Design review of the part built by this model. Coordinates are the model's own, in mm. Face numbers are marked on the shaded views. A direction names the side the tool comes from. Give positions to 0.01 mm unless a question says otherwise; leave off trailing zeros. Write each loop counter-clockwise with the first axis right and the second up, starting at its lowest first coordinate (ties: lowest second). Pieces come first, ordered by that corner, then holes.
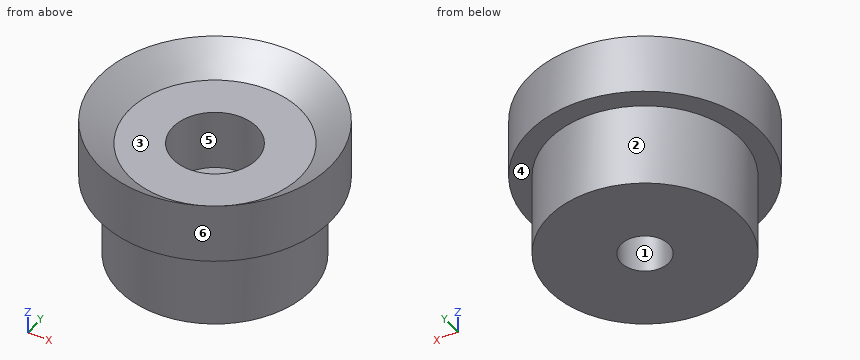
Autodesk Inventor part; units mm, degrees
ref_plane "YZ Plane" through (0, 0, 0) normal (1, 0, 0) x (0, 1, 0)
ref_plane "XZ Plane" through (0, 0, 0) normal (0, 1, 0) x (-1, 0, 0)
ref_plane "XY Plane" through (0, 0, 0) normal (0, 0, 1) x (1, 0, 0)
sketch "Sketch1" plane through (0, 0, 0) normal (1, 0, 0) x (0, 1, 0)
  line L0 (4.108, 9.9473) -> (-5.9746, 9.9473)
  line L1 (-5.9746, 9.9473) -> (-5.9746, 1.0479)
  line L2 (-5.9746, 1.0479) -> (-7.2571, 1.0479)
  line L3 (-7.2571, 1.0479) -> (-7.2571, -5.9277)
  line L4 (-7.2571, -5.9277) -> (5.4429, -5.9277)
  line L5 (5.4429, -5.9277) -> (5.4429, 5.1848)
  line L6 (5.4429, 5.1848) -> (8.0704, 5.1848)
  line L7 (8.0704, 5.1848) -> (8.0704, 13.1223)
  line L8 (4.108, 9.9473) -> (8.0704, 13.1223)
  line L9 (5.4429, -5.9277) -> (-46.9446, -5.9277) construction
  line L10 (-46.9446, -5.9277) -> (-46.9446, 28.5001)
  point P0 (0, 0)
  dimension "d3" = 19.05
  dimension "d4" = 7.9375
  dimension "d5" = 3.175
  dimension "d6" = 3.9624
  dimension "d7" = 12.7
  dimension "d20" = 52.3875
revolve "Revolution1" add sketch "Sketch1" angle 360 about axis through (0, -7.2571, 1.0479) along (0, 0, -1)
sketch "Sketch2" plane through (0, -7.2571, 9.9473) normal (0, 0, 1) x (1, 0, 0)
  circle A0 centre (0, 0) radius 1.2825
  circle A1 centre (0, 0) radius 5.5563
  point P0 (0, 7.2571)
  dimension "d9" = 11.1125
extrude "Extrusion1" cut sketch "Sketch2" against normal blind 7.9375
sketch "Sketch5" plane through (0, -7.2571, 2.0098) normal (0, 0, 1) x (1, 0, 0)
  circle A0 centre (0, 0) radius 3.175
  point P0 (0, 7.2571)
  dimension "d17" = 6.35
extrude "Extrusion4" cut sketch "Sketch5" against normal blind 211.1375
(1) Tool access review of the marked faces 1, 2 and 3: name each direction out of +Z, -Z, +X, -X, +Y, -Y from which nothing blocks a thin tool from reaching the whole face with its end or side.
Resolved:
face 1: +Z, -Z
face 2: -Z
face 3: +Z
(2) Consider section A-A, the plane x = 0. Give the boundary of the cut face in (y, z).
Resolved:
outline: (-22.58, 5.18) - (-19.96, 5.18) - (-19.96, -5.93) - (-10.43, -5.93) - (-10.43, 2.01) - (-12.81, 2.01) - (-12.81, 9.95) - (-18.62, 9.95) - (-22.58, 13.12) - close; (-4.08, -5.93) - (5.44, -5.93) - (5.44, 5.18) - (8.07, 5.18) - (8.07, 13.12) - (4.11, 9.95) - (-1.7, 9.95) - (-1.7, 2.01) - (-4.08, 2.01) - close
(3) Mouldability with a two-part tool opening along Y and no side actions: class the marked faces 4, 5 and 6 as pulls with the +Y half, pulls with the -Y half, needs draft (parallel to the pull), parting line crosses it, or undercut.
Resolved:
face 4: needs draft
face 5: undercut
face 6: parting line crosses it
(4) Consider section C-C, the plane z = 12. Give the boundary of the cut face in (x, y) (1 decimal).
Resolved:
outline: circle Ø30.7 at (0, -7.3); hole circle Ø27.9 at (0, -7.3)
(5) Consider section B-B, the plane z = 0. Give the boundary of the cut face in (x, y) (3 decimals), then the cut area to 3 significant figures.
Resolved:
outline: circle Ø25.4 at (0, -7.257); hole circle Ø6.35 at (0, -7.257)
area: 475 mm2
(6) To check wall thickness, follow L1, parallel to Z at x = -5, y = -9.5; L2, parallel to Z at x = 7, y = -13; L3, parallel to X at y = -9.5, z = 10.25. State the ranges of each line that lie inside material, in increasing order.
Resolved:
L1: z = -5.93 to 2.01
L2: z = -5.93 to 9.95
L3: x = -15.16 to -11.53, 11.53 to 15.16
(7) Clearance check with flat-ended pins moving along their axes: P1, Ø2, axis at x = 10.5, y = -10, coming from the +Z side; P2, Ø18, axis at x = 0, y = -7.26, coming from the +Z side; P3, Ø2, axis at y = -4, z = 1, coming from the -X side. State where each tip first meets the part, or that it passes through.
Resolved:
P1: stops at z = 10.34
P2: stops at z = 9.95
P3: stops at x = -12.5
